For this review, take the finished solid that the model builds, in its own axes (mm). Face numbers are marked on the shaded views. A direction names the side the tool comes from. Give positions to 0.01 mm unless a question says otherwise; leave off trailing zeros. Write each loop counter-clockwise with the first axis right and the second up, starting at its lowest first coordinate (ties: lowest second). Pieces come first, ordered by that corner, then holes. Notation, with made-up numbers: (66.5, 65.5) -> (95.5, 65.5) arc R22 ccw to (95.5, 83.5) -> close; hole circle Ø3 at (-32, 23). An arc over 180 degrees is marked (long way). Answer as CSV lines item,"result".
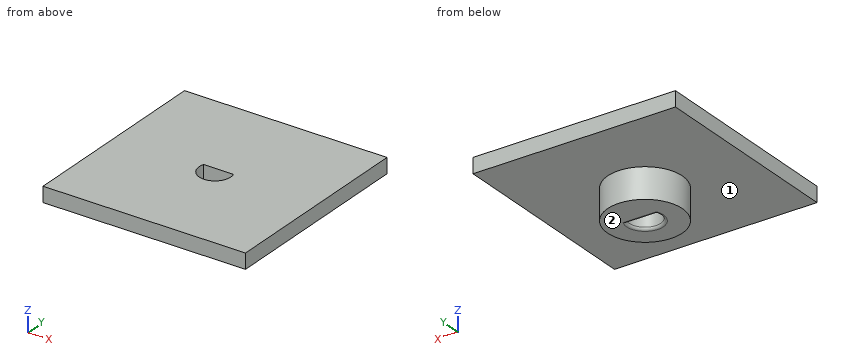
Autodesk Inventor part; units mm, degrees
ref_plane "YZ Plane" through (0, 0, 0) normal (1, 0, 0) x (0, 1, 0)
ref_plane "XZ Plane" through (0, 0, 0) normal (0, 1, 0) x (-1, 0, 0)
ref_plane "XY Plane" through (0, 0, 0) normal (0, 0, 1) x (1, 0, 0)
sketch "Sketch8" plane through (0, 0, 0) normal (0, 0, 1) x (1, 0, 0)
  line L0 (0, 0) -> (40, 0)
  line L1 (40, 0) -> (40, 40)
  line L2 (40, 40) -> (0, 40)
  line L3 (0, 40) -> (0, 0)
  dimension "d35" = 40
  dimension "d36" = 40
extrude "Extrusion8" add sketch "Sketch8" along normal blind 3
sketch "Sketch9" plane through (0, 0, 0) normal (0, 0, -1) x (-1, 0, 0)
  line L0 (0, 40) -> (0, 0)
  line L1 (0, 20) -> (-20, 20)
  circle A0 centre (-20, 20) radius 7.375
  dimension "d39" = 20
  dimension "d40" = 14.75
extrude "Extrusion9" add sketch "Sketch9" along normal blind 6
sketch "Sketch10" plane through (20, 20, -6) normal (0, 0, -1) x (-1, 0, 0)
  circle A0 centre (0, 0) radius 3.125
  line L0 (0, 0) -> (0, 1)
  line L1 (0, 1) -> (-2.9607, 1)
  line L2 (0, 1) -> (2.9607, 1)
  point P0 (20, -20)
  dimension "d43" = 6.25
  dimension "d44" = 1
extrude "Extrusion10" cut sketch "Sketch10" against normal up to next contours A0 L1 L2 picked at (-0.0807, -1.7325)
fillet "Fillet1" radius 0.5 2 edges at (20, 16.875, -6) (20, 21, -6)
equation "\"BendRadius\" = Thickness"
equation "\"BendReliefWidth\" = Thickness"
equation "\"BendReliefDepth\" = 0.5 * Thickness"
equation "\"CornerReliefSize\" = 4 * Thickness"
equation "\"MinimumRemnant\" = 2 * Thickness"
equation "\"TransitionRadius\" = BendRadius"
equation "\"JacobiRadiusSize\" = BendRadius"
equation "\"GapSize\" = Thickness"
properties part number "baseRotor1"
Q1. Add section A-A (y = 20). Write out the cut boundary in (x, z) (3 decimals).
Answer block:
outline,"(0, 0) -> (12.625, 0) -> (12.625, -6) -> (16.375, -6) arc R0.5 ccw to (16.875, -5.5) -> (16.875, 3) -> (0, 3) -> close; (23.125, -5.5) arc R0.5 ccw to (23.625, -6) -> (27.375, -6) -> (27.375, 0) -> (40, 0) -> (40, 3) -> (23.125, 3) -> close"
Q2. Add section B-B (x = 20). Write out the cut boundary in (y, z) (3 decimals).
Answer block:
outline,"(0, 0) -> (12.625, 0) -> (12.625, -6) -> (16.375, -6) arc R0.5 ccw to (16.875, -5.5) -> (16.875, 3) -> (0, 3) -> close; (21, -5.5) arc R0.5 ccw to (21.5, -6) -> (27.375, -6) -> (27.375, 0) -> (40, 0) -> (40, 3) -> (21, 3) -> close"
Q3. To check wall thickness, follow probe 1 along Y at (x, z) = (20, 0.25) (3 decimals); probe 2 along X at (y, z) = (20, 1.25) (3 decimals); probe 3 along Y at (x, z) = (20, -1.5) (3 decimals). State the ranges of each line that lie inside material, in increasing order. Write a range as [from, to].
Answer block:
probe 1,"y = [0, 16.875], [21, 40]"
probe 2,"x = [0, 16.875], [23.125, 40]"
probe 3,"y = [12.625, 16.875], [21, 27.375]"
Q4. Add section D-D (y = 33). Write out the cut boundary in (x, z), plus the area to 3 significant figures.
Answer block:
outline,"(0, 0) -> (40, 0) -> (40, 3) -> (0, 3) -> close"
area,"120 mm2"
Q5. Add section C-C (x = 15.5). Write out the cut boundary in (y, z).
Answer block:
outline,"(0, 0) -> (14.16, 0) -> (14.16, -6) -> (25.84, -6) -> (25.84, 0) -> (40, 0) -> (40, 3) -> (0, 3) -> close"
Q6. Clearance check with flat-ended pins moving along their axes: pin 1 (1 mm diameter, centred on y = 28.5, z = -1.5, fed in from +X); pin 2 (1 mm diameter, centred on x = 7, y = 10, fed in from -Z); pin 3 (4 mm diameter, centred on y = 26.5, z = -4, fed in from +X). State where each tip first meets the part, or that it passes through.
Answer block:
pin 1,"passes through"
pin 2,"stops at z = 0"
pin 3,"stops at x = 25.84"
Q7. For the marked faces 1 and 2, list the 3-axis set-ups (+Z, -Z, +X, -X, +Y, -Y) from which the entire face can be reached by the end or side of a thin tool; tool diameter is ignored.
Answer block:
face 1,"-Z"
face 2,"-Z, +X, -X, +Y, -Y"
